from build123d import *

# Parameters (mm, degrees)
SKETCH1_W                = 16.5862
SKETCH1_H                = 13.7922
BOSS_EXTRUDE1_DEPTH      = 9.144
SKETCH2_R                = 1.27
BOSS_EXTRUDE2_DEPTH      = 7.874
BOSS_EXTRUDE2_DEPTH_BACK = 6.096


with BuildPart() as part:
    # Sketch1 → Boss-Extrude1 (new body)
    with BuildSketch(Plane(origin=(0, 0, 0), x_dir=(1, 0, 0), z_dir=(0, 1, 0))):
        Rectangle(SKETCH1_W, SKETCH1_H)
    extrude(amount=BOSS_EXTRUDE1_DEPTH)

    # Sketch2 → Boss-Extrude2 (add, two sides)
    with BuildSketch(Plane(origin=(8.2931, 0, 0), x_dir=(0, 0, -1), z_dir=(1, 0, 0))) as boss_extrude2_sk:
        with Locations((0, 1.524)):
            Circle(SKETCH2_R)
        with Locations((-4.3561, 9.906)):
            Circle(SKETCH2_R)
    extrude(amount=BOSS_EXTRUDE2_DEPTH)
    extrude(boss_extrude2_sk.sketch, amount=-BOSS_EXTRUDE2_DEPTH_BACK)


solid = part.part
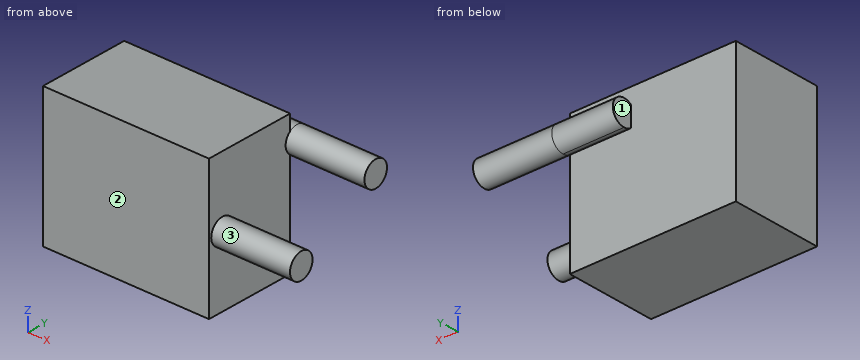
Could you check a few things on this model? Use its own coordinates, in mm. Face numbers are marked on the shaded views. A direction names the side the tool comes from. Give positions to 0.01 mm unless a question says otherwise; leave off trailing zeros. Loops run counter-clockwise (first coordinate to the right, second up) from the corner with the lowest first, then second, coordinate; pieces in that order, holes last. Notation, with made-up numbers: M -26.75,75.25 L -17.75,75.25 A36 ccw -17.75,112.25 Z; hole C -10.5,25.25 d5. An arc over 180 degrees is marked long. Answer as a JSON object with one key per item and string values.
Q1. Suppose I cut it at B-B, the plane x = 14. List the corners of the cut face in (y, z) for me.
Values found:
{"outline": "C 1.52,0 d2.54; C 9.91,4.36 d2.54"}
Q2. Suppose I cut it at D-D, the plane x = 6.5. List the corners of the cut face in (y, z) for me.
Values found:
{"outline": "M 0,-6.9 L 9.14,-6.9 L 9.14,3.34 A1.27 ccw long 9.14,5.37 L 9.14,6.9 L 0,6.9 Z"}
Q3. Suppose I cut it at A-A, the plane z = 0. List the corners of the cut face in (x, y) for me, plus the area to 3 significant figures.
Values found:
{"outline": "M -8.29,0 L 8.29,0 L 8.29,0.25 L 16.17,0.25 L 16.17,2.79 L 8.29,2.79 L 8.29,9.14 L -8.29,9.14 Z", "area": "172 mm²"}
Q4. For P1, Ø1.5, axis at y = 8, z = 5.5, coming from the +X side; P2, Ø1, axis at x = 9.5, y = 8.5, coming from the -Z side; P3, Ø1, axis at x = 10.5, y = 9, coming from the +Z side, each with a flat end and sliding along its axis, tell me the tip position at first contact or that it passes through.
Values found:
{"P1": "stops at x = 8.29", "P2": "stops at z = 3.47", "P3": "stops at z = 5.56"}
Q5. For the marked faces 1, 2 and 3, which set-ups out of +Z, -Z, +X, -X, +Y, -Y let a thin tool reach every point of the face, with its end or its side?
Values found:
{"face 1": "+Z, -Z, -X, +Y", "face 2": "+Z, -Z, +X, -X, -Y", "face 3": "+X"}
Q6. If I drill on probe 1 along Y at (x, z) = (-5.75, 4); probe 2 along Y at (x, z) = (12.5, 0); probe 3 along X at (y, z) = (7.5, -0.5), over which ranges is the centre line in solid material (lowest first)? Write a range as [from, to].
Values found:
{"probe 1": "y = [0, 9.14]", "probe 2": "y = [0.25, 2.79]", "probe 3": "x = [-8.29, 8.29]"}
Q7. Suppose I cut it at C-C, the plane y = 5. List the corners of the cut face in (x, z) for me, plus the area to 3 significant figures.
Values found:
{"outline": "M -8.29,-6.9 L 8.29,-6.9 L 8.29,6.9 L -8.29,6.9 Z", "area": "229 mm²"}
